```python
from build123d import *

# Parameters (mm, degrees)
F0_R     = 24
F1_DEPTH = 12
F2_R     = 5
F3_R     = 17
F4_DEPTH = 10


with BuildPart() as f1:
    # F0 (on Top) → F1 (new body)
    with BuildSketch(Plane.XY):
        Circle(F0_R)
    extrude(amount=F1_DEPTH)

    # F2
    f2_edges = [f1.edges().sort_by_distance(p)[0] for p in [
        (-24, 0, 12),
    ]]
    fillet(f2_edges, radius=F2_R)

    # F3 (on face) → F4 (cut)
    with BuildSketch(Plane.XY.offset(12)):
        Circle(F3_R)
    extrude(amount=-F4_DEPTH, mode=Mode.SUBTRACT)


solid = f1.part
```
The listing builds one solid part. Answer for the finished solid, in the listing's coordinates (mm). A direction names the side the tool comes from. Give positions to 0.01 mm unless a question says otherwise; leave off trailing zeros. Loops run counter-clockwise (first coordinate to the right, second up) from the corner with the lowest first, then second, coordinate; pieces in that order, holes last. Notation, with made-up numbers: M 10,0 L 61,0 A22 cw 61,37 Z; hole C 23,-9 d10. An arc over 180 degrees is marked long. One line per item, written item: value.
Q1. Determine the mould class of faces 1 (the face through (-23.977, 1.055, 3.451)), 2 (the face through (0, 0, 2)), 3 (the face through (-14, -10, 12)) for opening direction X: +X half, -X half, draft (parallel to the pull), parting line (faces both ways), or undercut.
Working result:
face 1: parting line
face 2: undercut
face 3: draft
Q2. A cutting plane is placed at D-D on z = 7.75. Determine the outline of the cut face in (x, y).
Working result:
outline: C 0,0 d47.89; hole C 0,0 d34
Q3. Flat-ended cylindrical pins translate along their axes: P1, Ø1.5, axis at y = -2.5, z = 8, coming from the -X side; P2, Ø5, axis at x = -15, z = 3, coming from the -Y side; P3, Ø1, axis at x = 16, y = -16.5, coming from the +Z side. Find the tip coordinate at first contact, or state that the pin passes through.
Working result:
P1: stops at x = -23.9
P2: stops at y = -20.49
P3: stops at z = 10.59
Q4. A cutting plane is placed at C-C on z = 1.25. Determine the outline of the cut face in (x, y).
Working result:
outline: C 0,0 d48
Q5. For faces 4 (the face through (9.139, 14.334, 7.07)), 5 (the face through (0, 0, 0)), determine the directions among +Z, -Z, +X, -X, +Y, -Y from which every point of the face is accessible in a straight line to the end or side of a thin tool.
Working result:
face 4: +Z
face 5: -Z, +X, -X, +Y, -Y
Q6. Find the intervals of material crossed by line 1 (Y direction, x = 0, z = 6.75); line 2 (Z direction, x = -5, y = -1.5); line 3 (Y direction, x = -12, z = 4), in increasing order. Write a range as from..to.
Working result:
line 1: y = -24..-17, 17..24
line 2: z = 0..2
line 3: y = -20.78..-12.04, 12.04..20.78
Q7. A cutting plane is placed at A-A on x = 0. Determine the outline of the cut face in (y, z).
Working result:
outline: M -24,0 L 24,0 L 24,7 A5 ccw 19,12 L 17,12 L 17,2 L -17,2 L -17,12 L -19,12 A5 ccw -24,7 Z
